from build123d import *

# Parameters (mm, degrees)
BOSS_EXTRUDE1_DEPTH = 18
CUT_EXTRUDE1_START  = -2.5
CUT_EXTRUDE1_DEPTH  = 13
CUT_EXTRUDE2_START  = -2.5
CUT_EXTRUDE2_DEPTH  = 13
SKETCH5_R           = 1
SKETCH5_R_2         = 1.5
CUT_EXTRUDE3_DEPTH  = 25
FILLET1_R           = 3


with BuildPart() as part:
    # Sketch2 → Boss-Extrude1 (new body)
    with BuildSketch(Plane.XY):
        with BuildLine():
            Line((0, 0), (12, 0))
            Line((12, 0), (17.171830748, 6.163547874))
            ThreePointArc((17.171830748, 6.163547874), (17.692775281, 7.065850273), (17.873697418, 8.091910703))
            Line((17.873697418, 8.091910703), (17.873697418, 17.672459688))
            ThreePointArc((17.873697418, 17.672459688), (17.592620779, 18.940314473), (16.802060247, 19.970593018))
            Line((16.802060247, 19.970593018), (12, 24))
            Line((12, 24), (2, 24))
            Line((2, 24), (0, 0))
        make_face()
    extrude(amount=BOSS_EXTRUDE1_DEPTH)

    # Sketch3 → Cut-Extrude1 (cut)
    with BuildSketch(Plane.XY.offset(18).offset(CUT_EXTRUDE1_START)):
        with BuildLine():
            Line((7, 24), (9, 24))
            Line((9, 24), (9, 22.791287847))
            ThreePointArc((9, 22.791287847), (8, 18), (7, 22.791287847))
            Line((7, 22.791287847), (7, 24))
        make_face()
    extrude(amount=-CUT_EXTRUDE1_DEPTH, mode=Mode.SUBTRACT)

    # Sketch4 → Cut-Extrude2 (cut)
    with BuildSketch(Plane(origin=(0, 0, 0), x_dir=(-1, 0, 0), z_dir=(0, 0, -1)).offset(CUT_EXTRUDE2_START)):
        with BuildLine():
            Line((-9, 0), (-7, 0))
            Line((-7, 0), (-7, 1.208712153))
            ThreePointArc((-7, 1.208712153), (-8, 6), (-9, 1.208712153))
            Line((-9, 1.208712153), (-9, 0))
        make_face()
    extrude(amount=-CUT_EXTRUDE2_DEPTH, mode=Mode.SUBTRACT)

    # Sketch5 → Cut-Extrude3 (cut)
    with BuildSketch(Plane(origin=(0, 0, 0), x_dir=(1, 0, 0), z_dir=(0, 1, 0))):
        with Locations((15, -9)):
            Circle(SKETCH5_R)
        with Locations((15, -13)):
            Circle(SKETCH5_R_2)
    extrude(amount=CUT_EXTRUDE3_DEPTH, mode=Mode.SUBTRACT)

    # Fillet1
    fillet1_edges = [part.edges().sort_by_distance(p)[0] for p in [
        (17.692775281, 7.065850273, 0),
        (14.585915374, 3.081773937, 0),
        (1, 12, 0),
        (14.585915374, 3.081773937, 18),
        (17.692775281, 7.065850273, 18),
        (17.873697418, 12.882185196, 18),
        (17.592620779, 18.940314473, 18),
        (14.401030124, 21.985296509, 18),
        (1, 12, 18),
        (14.401030124, 21.985296509, 0),
        (17.592620779, 18.940314473, 0),
        (17.873697418, 12.882185196, 0),
    ]]
    fillet(fillet1_edges, radius=FILLET1_R)


solid = part.part
The listing builds one solid part. Answer for the finished solid, in the listing's coordinates (mm). A direction names the side the tool comes from. Give positions to 0.01 mm unless a question says otherwise; leave off trailing zeros. Write each loop counter-clockwise with the first axis right and the second up, starting at its lowest first coordinate (ties: lowest second). Pieces come first, ordered by that corner, then holes. Notation, with made-up numbers: (-30.75, -28) -> (-5.75, -28) arc R20 ccw to (-5.75, 9) -> close; hole circle Ø6 at (-6, 39.5). An arc over 180 degrees is marked (long way). One line per question, with ' | ' between items. Start each with the question number.
1. Section B-B (z = 11) is taken. Determine the outline of the cut face in (x, y), plus the area to 3 significant figures.
2. Given pin 1 Ø3 at (y, z) = (7.5, 6) entering from -X; pin 2 Ø1.3 at (y, z) = (23.5, 6) entering from -X; pin 3 Ø5 at (x, z) = (15, 13) entering from -Y, each flat-ended and moving along its own axis, determine where each tip first touches the part or whether it passes through.
3. For a pull along Y with two mould halves and no side action, classify faces 1 (the cylindrical face through (16.972, 12.949, 0.855)), 2 (the cylindrical face through (1.85, 11.88, 0.9)), 3 (the cylindrical face through (8, 18, 9)), 4 (the cylindrical face through (13.89, 3.65, 17.14)) as pulls with the +Y half, pulls with the -Y half, needs draft (parallel to the pull), parting line crosses it, or undercut.
4. Section A-A (z = 9) is taken. Determine the outline of the cut face in (x, y), plus the area to 3 significant figures.
5. Find the intervals of material crossed by probe 1 along Z at (x, y) = (15, 12.75); probe 2 along Y at (x, z) = (6.5, 7.75); probe 3 along Z at (x, y) = (15.75, 7.5), in increasing order.
6. Section D-D (z = 16) is taken. Determine the outline of the cut face in (x, y), plus the area to 3 significant figures.
7. Section C-C (y = 14) is taken. State how many separate pieces and enclosed holes the cut face has, plus the area to 3 significant figures.
8. For faces 5 (the flat face through (8, 21, 15.5)), 6 (the flat face through (1, 12, 9)), 7 (the flat face through (9, 1, 9)), 8 (the flat face through (9, 23, 9)), determine the directions among +Z, -Z, +X, -X, +Y, -Y from which every point of the face is accessible in a straight line to the end or side of a thin tool.
Response values:
1) outline: (0, 0) -> (7, 0) -> (7, 1.21) arc R2.5 cw (long way) to (9, 1.21) -> (9, 0) -> (12, 0) -> (17.17, 6.16) arc R3 ccw to (17.87, 8.09) -> (17.87, 17.67) arc R3 ccw to (16.8, 19.97) -> (12, 24) -> (9, 24) -> (9, 22.79) arc R2.5 cw (long way) to (7, 22.79) -> (7, 24) -> (2, 24) -> close | area: 326 mm2
2) pin 1: x = 0.5 | pin 2: x = 1.9 | pin 3: y = 0.6
3) face 1: needs draft | face 2: pulls with the +Y half | face 3: undercut | face 4: pulls with the -Y half
4) outline: (0, 0) -> (7, 0) -> (7, 1.21) arc R2.5 cw (long way) to (9, 1.21) -> (9, 0) -> (12, 0) -> (14, 2.38) -> (14, 22.32) -> (12, 24) -> (9, 24) -> (9, 22.79) arc R2.5 cw (long way) to (7, 22.79) -> (7, 24) -> (2, 24) -> close; (16, 4.77) -> (17.17, 6.16) arc R3 ccw to (17.87, 8.09) -> (17.87, 17.67) arc R3 ccw to (16.8, 19.97) -> (16, 20.64) -> close | area: 290 mm2
5) probe 1: 0 to 8, 10 to 11.5, 14.5 to 18 | probe 2: 0 to 1.5, 5.5 to 18.5, 22.5 to 24 | probe 3: 0.19 to 8.34, 9.66 to 11.7, 14.3 to 17.81
6) outline: (0.17, 0) -> (11.78, 0) -> (17.04, 6.27) arc R2.83 ccw to (17.7, 8.09) -> (17.7, 17.67) arc R2.83 ccw to (16.69, 19.84) -> (11.73, 24) -> (2.17, 24) -> close | area: 360 mm2
7) separate pieces: 1 | enclosed holes: 2 | area: 283 mm2
8) face 5: none | face 6: +Z, -Z, -X, +Y | face 7: -Y | face 8: +Y
